```python
from build123d import *

# Parameters (mm, degrees)
BOSS_EXTRUDE1_DEPTH = 45.72
SKETCH2_R           = 2.032
CUT_EXTRUDE1_DEPTH  = 45.72


with BuildPart() as part:
    # Sketch1 → Boss-Extrude1 (new body)
    with BuildSketch(Plane.XY):
        Polygon((-3.175, 0.884089911), (-3.175, 3.175), (-0.979194969, 3.175), (-0.979194969, 28.575), (0.978019253, 28.575), (0.978019253, 3.175), (3.175, 3.175), (3.175, 0.884089911), (28.575, 0.884089911), (28.575, -0.86253999), (3.175, -0.86253999), (3.175, -3.175), (0.978019253, -3.175), (0.978019253, -28.575), (-0.979194969, -28.575), (-0.979194969, -3.175), (-3.175, -3.175), (-3.175, -0.86253999), (-28.575, -0.86253999), (-28.575, 0.884089911), align=None)
    extrude(amount=BOSS_EXTRUDE1_DEPTH)

    # Sketch2 → Cut-Extrude1 (cut)
    with BuildSketch(Plane.XY.offset(45.72)):
        Circle(SKETCH2_R)
    extrude(amount=-CUT_EXTRUDE1_DEPTH, mode=Mode.SUBTRACT)


solid = part.part
```
Design review of the part built by this model. Coordinates are the model's own, in mm. A direction names the side the tool comes from. Give positions to 0.01 mm unless a question says otherwise; leave off trailing zeros. Write each loop counter-clockwise with the first axis right and the second up, starting at its lowest first coordinate (ties: lowest second). Pieces come first, ordered by that corner, then holes.
(1) Wall thickness on line 1 along X through (y, z) = (-17.5, 19.5); line 2 along Y through (x, z) = (0, 14) (3 decimals); line 3 along Y through (x, z) = (-12, 28): over which ranges is each line inside the solid? List them lowest first.
Checked values:
line 1: x = -0.98 to 0.98
line 2: y = -28.575 to -2.032, 2.032 to 28.575
line 3: y = -0.86 to 0.88
(2) Clearance check with flat-ended pins moving along their axes: pin 1 Ø0.7 at (y, z) = (-2.5, 20) entering from -X (3 decimals); pin 2 Ø4 at (x, z) = (5, 5) entering from +Y (3 decimals); pin 3 Ø3.5 at (x, y) = (0, 0) entering from -Z; pin 4 Ø20.5 at (x, z) = (16.5, 23.5) entering from -Y. State where each tip first meets the part, or that it passes through.
Checked values:
pin 1: stops at x = -3.175
pin 2: stops at y = 3.175
pin 3: passes through
pin 4: stops at y = -0.86
(3) Add section C-C (z = 35). Give the boundary of the cut face in (x, y) (3 decimals).
Checked values:
outline: (-28.575, -0.863) - (-3.175, -0.863) - (-3.175, -3.175) - (-0.979, -3.175) - (-0.979, -28.575) - (0.978, -28.575) - (0.978, -3.175) - (3.175, -3.175) - (3.175, -0.863) - (28.575, -0.863) - (28.575, 0.884) - (3.175, 0.884) - (3.175, 3.175) - (0.978, 3.175) - (0.978, 28.575) - (-0.979, 28.575) - (-0.979, 3.175) - (-3.175, 3.175) - (-3.175, 0.884) - (-28.575, 0.884) - close; hole circle Ø4.064 at (0, 0)
(4) Mouldability with a two-part tool opening along Y and no side actions: class faces 1 (the face through (-3.175, -2, 23)), 2 (the face through (0, 28.575, 23)), 3 (the face through (-0.44, -1.984, 23.18)) as +Y half, -Y half, draft (parallel to the pull), parting line (faces both ways), or undercut.
Checked values:
face 1: draft
face 2: +Y half
face 3: undercut
(5) Add section A-A (y = 0). Give the boundary of the cut face in (x, z) (3 decimals).
Checked values:
outline: (-28.575, 0) - (-2.032, 0) - (-2.032, 45.72) - (-28.575, 45.72) - close; (2.032, 0) - (28.575, 0) - (28.575, 45.72) - (2.032, 45.72) - close
(6) Tool access review of faces 4 (the face through (-0.979, -16, 23)), 5 (the face through (16, 0.884, 23)), 6 (the face through (-0.979, 16, 23)), 7 (the face through (3.175, -2, 23)): name each direction out of +Z, -Z, +X, -X, +Y, -Y from which nothing blocks a thin tool from reaching the whole face with its end or side.
Checked values:
face 4: +Z, -Z, -X, -Y
face 5: +Z, -Z, +X, +Y
face 6: +Z, -Z, -X, +Y
face 7: +Z, -Z, +X, -Y
(7) Add section D-D (x = -13). Give the boundary of the cut face in (y, z).
Checked values:
outline: (-0.86, 0) - (0.88, 0) - (0.88, 45.72) - (-0.86, 45.72) - close
